Verification items for this drawing (mm, ordinates from the low corner). A direction names the side the tool comes from. Give positions to 0.01 mm unless a question says otherwise; leave off trailing zeros. Order: outer loops, then holes, each group sorted by start corner. A loop starts at its lowest first (then second) coordinate and runs counter-clockwise, first axis right, second up. Notation, with made-up numbers: (31.5, 69) -> (71.5, 69) arc R22 cw to (71.5, 98) -> close; hole circle Ø2 at (83.5, 68.5). An arc over 180 degrees is marked (long way). One line per question, with ' | ' between items.
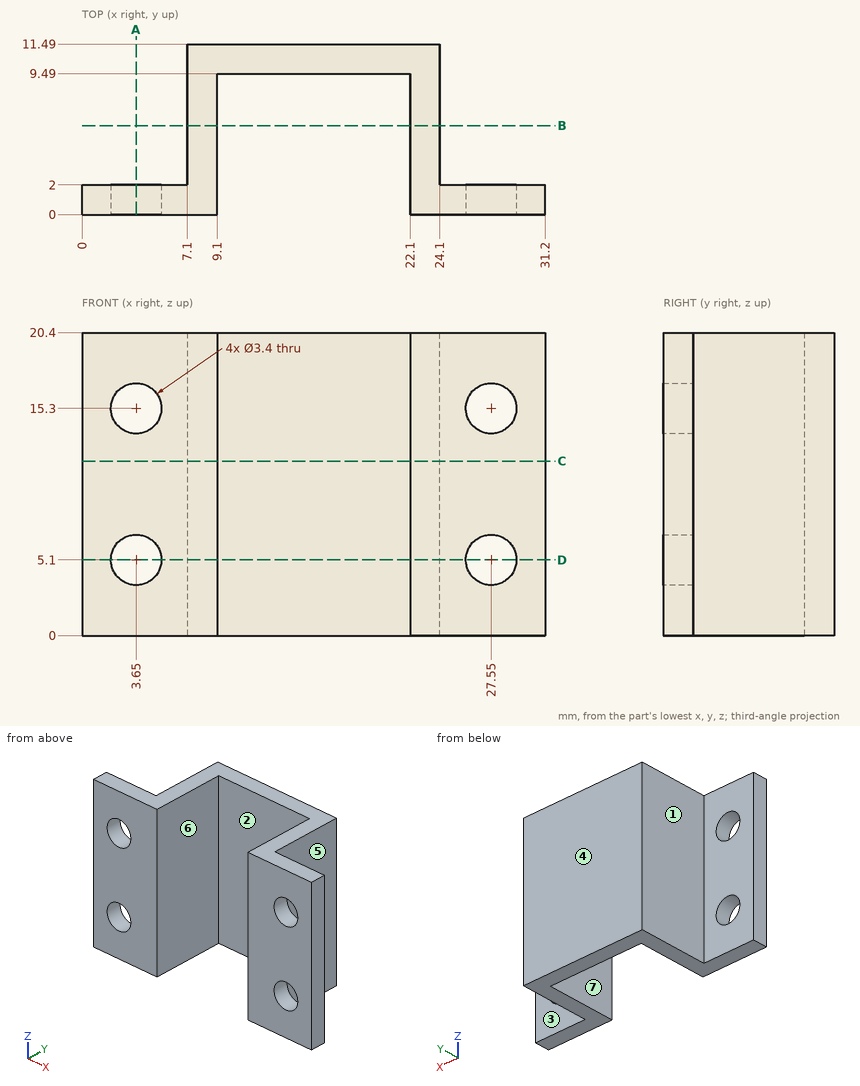
Q1. Depth check by flat-ended pin: pin 1 Ø10.5 at (x, z) = (15.5, 8.5) entering from -Y; pin 2 Ø4.5 at (y, z) = (6.5, 13) entering from +X; pin 3 Ø3 at (y, z) = (8.5, 7.5) entering from -X; pin 4 Ø2 at (x, z) = (3.65, 15.3) entering from +Y. Enter the tip coordinate at first touch or a pass-through.
Result sheet:
pin 1: stops at y = 9.49 | pin 2: stops at x = 24.1 | pin 3: stops at x = 7.1 | pin 4: passes through
Q2. Access from +Z, -Z, +X, -X, +Y, -Y to the whole of each face (thin tool, end or side, straight path). Record for the marked faces 1, 2 and 3.
Result sheet:
face 1: +Z, -Z, -X, +Y | face 2: +Z, -Z, -Y | face 3: +Z, -Z, +X, +Y
Q3. Section check A-A (x = 3.65). Enter the section's corners in (y, z), and give its area (3 significant figures).
Result sheet:
outline: (0, 0) -> (2, 0) -> (2, 3.4) -> (0, 3.4) -> close; (0, 6.8) -> (2, 6.8) -> (2, 13.6) -> (0, 13.6) -> close; (0, 17) -> (2, 17) -> (2, 20.4) -> (0, 20.4) -> close | area: 27.2 mm2
Q4. Thickness scan on line 1 (X direction, y = 1.35, z = 5.1); line 2 (X direction, y = 3.5, z = 6.75); line 3 (X direction, y = 1.5, z = 14.25). Record the ranges inside material, lowest first.
Result sheet:
line 1: x = 0 to 1.95, 5.35 to 9.1, 22.1 to 25.85, 29.25 to 31.2 | line 2: x = 7.1 to 9.1, 22.1 to 24.1 | line 3: x = 0 to 2.31, 4.99 to 9.1, 22.1 to 26.21, 28.89 to 31.2
Q5. Section check D-D (z = 5.1). Enter the section's corners in (x, y).
Result sheet:
outline: (0, 0) -> (1.95, 0) -> (1.95, 2) -> (0, 2) -> close; (5.35, 0) -> (9.1, 0) -> (9.1, 9.49) -> (22.1, 9.49) -> (22.1, 0) -> (25.85, 0) -> (25.85, 2) -> (24.1, 2) -> (24.1, 11.49) -> (7.1, 11.49) -> (7.1, 2) -> (5.35, 2) -> close; (29.25, 0) -> (31.2, 0) -> (31.2, 2) -> (29.25, 2) -> close
Q6. Section check C-C (z = 11.75). Enter the section's corners in (x, y), and give its area (3 significant figures).
Result sheet:
outline: (0, 0) -> (9.1, 0) -> (9.1, 9.49) -> (22.1, 9.49) -> (22.1, 0) -> (31.2, 0) -> (31.2, 2) -> (24.1, 2) -> (24.1, 11.49) -> (7.1, 11.49) -> (7.1, 2) -> (0, 2) -> close | area: 100 mm2
Q7. Section check B-B (y = 6). Enter the section's corners in (x, z), and give its area (3 significant figures).
Result sheet:
outline: (7.1, 0) -> (9.1, 0) -> (9.1, 20.4) -> (7.1, 20.4) -> close; (22.1, 0) -> (24.1, 0) -> (24.1, 20.4) -> (22.1, 20.4) -> close | area: 81.6 mm2
Q8. Mould release check, pull along X, two halves, no side actions. Record for the marked faces 4, 5, 6 and 7: pulls with the +X half, pulls with the -X half, needs draft (parallel to the pull), parting line crosses it, or undercut.
Result sheet:
face 4: needs draft | face 5: pulls with the +X half | face 6: undercut | face 7: undercut
